Drawing for the job (mm, zero at the part's lowest x, y, z). A direction names the side the tool comes from. Round coordinates to 2 decimals unless told otherwise and drop trailing zeros. Order: outer loops, then holes, each group sorted by start corner. A loop starts at its lowest first (then second) coordinate and runs counter-clockwise, first axis right, second up. Notation, with made-up numbers: (55, 68) - (61, 68) arc R14 ccw to (61, 84) - close; hole circle Ø9 at (-40, -35.75). An arc over 180 degrees is marked (long way). Put each result on its own line as item: value. Start each with the question number.
Item 1: Probe probe 1 along Z at (x, y) = (26, 5.35); probe 2 along Z at (x, y) = (48.5, 4.6); probe 3 along X at (y, z) = (4.75, 14.5). List the from-to ranges inside material, lowest first.
Item 2: Mould opens along X. For the marked faces 3, 4 and 5 say: pulls with the +X half, pulls with the -X half, needs draft (parallel to the pull), parting line crosses it, or undercut.
Item 3: Saw through at C-C on z = 13.5. List the corners of the cut face in (x, y).
Item 4: Which spindle directions (+Z, -Z, +X, -X, +Y, -Y) get a long thin tool onto all of the face, cutting with end or side? Do the marked faces 1 and 2. Say none if no direction does.
Item 5: Saw through at B-B on z = 10.5. List the corners of the cut face in (x, y).
Item 6: Saw through at A-A on x = 48.5. List the corners of the cut face in (y, z), plus the area to 3 significant figures.
Item 7: Pin check, flat tips, straight feed: pin 1 Ø7 at (x, z) = (8.5, 10.5) entering from +Y; pin 2 Ø5 at (x, z) = (30, 6) entering from -Y. Stop position of each tip, or through.
Item 8: Saw through at D-D on y = 0.95. List the corners of the cut face in (x, z).
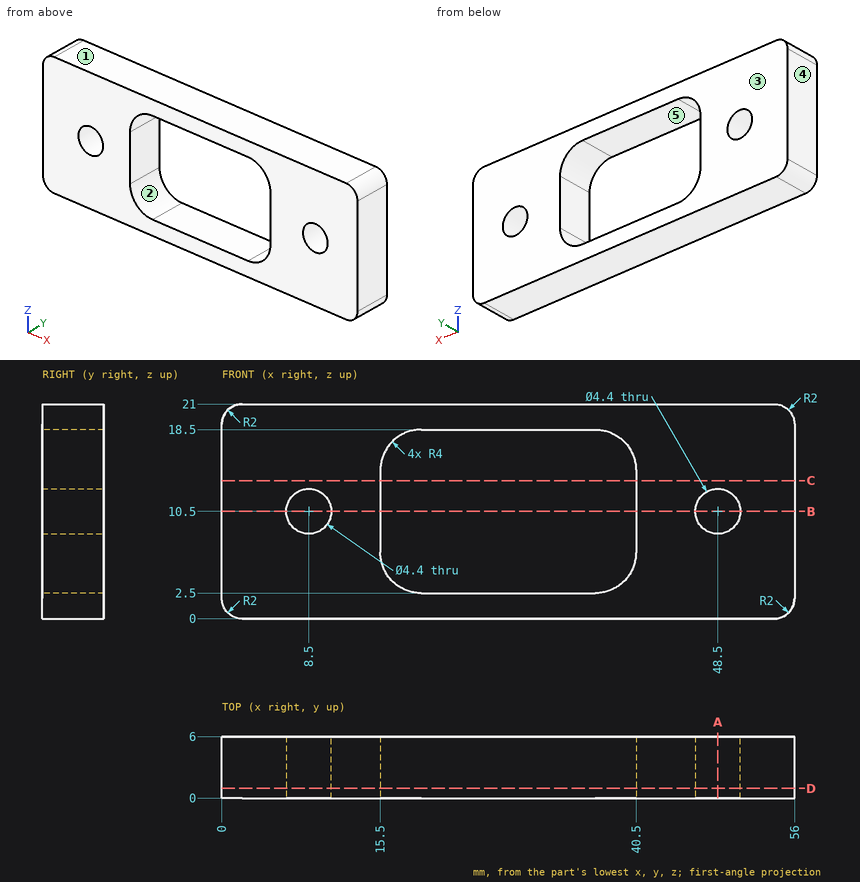
Results found:
1. probe 1: z = 0 to 2.5, 18.5 to 21
1. probe 2: z = 0 to 8.3, 12.7 to 21
1. probe 3: x = 0 to 15.5, 40.5 to 56
2. face 3: needs draft
2. face 4: pulls with the -X half
2. face 5: undercut
3. outline: (0, 0) - (15.5, 0) - (15.5, 6) - (0, 6) - close; (40.5, 0) - (56, 0) - (56, 6) - (40.5, 6) - close
4. face 1: +Z, +X, -X, +Y, -Y
4. face 2: +Y, -Y
5. outline: (0, 0) - (6.3, 0) - (6.3, 6) - (0, 6) - close; (10.7, 0) - (15.5, 0) - (15.5, 6) - (10.7, 6) - close; (40.5, 0) - (46.3, 0) - (46.3, 6) - (40.5, 6) - close; (50.7, 0) - (56, 0) - (56, 6) - (50.7, 6) - close
6. outline: (0, 0) - (6, 0) - (6, 8.3) - (0, 8.3) - close; (0, 12.7) - (6, 12.7) - (6, 21) - (0, 21) - close
6. area: 99.6 mm²
7. pin 1: stops at y = 6
7. pin 2: passes through
8. outline: (0, 2) arc R2 ccw to (2, 0) - (54, 0) arc R2 ccw to (56, 2) - (56, 19) arc R2 ccw to (54, 21) - (2, 21) arc R2 ccw to (0, 19) - close; hole circle Ø4.4 at (8.5, 10.5); hole (15.5, 6.5) arc R4 ccw to (19.5, 2.5) - (36.5, 2.5) arc R4 ccw to (40.5, 6.5) - (40.5, 14.5) arc R4 ccw to (36.5, 18.5) - (19.5, 18.5) arc R4 ccw to (15.5, 14.5) - close; hole circle Ø4.4 at (48.5, 10.5)
